Autodesk Inventor part; units mm, degrees
ref_plane "YZ Plane" through (0, 0, 0) normal (1, 0, 0) x (0, 1, 0)
ref_plane "XZ Plane" through (0, 0, 0) normal (0, 1, 0) x (-1, 0, 0)
ref_plane "XY Plane" through (0, 0, 0) normal (0, 0, 1) x (1, 0, 0)
sketch "Sketch1" plane through (0, 0, 0) normal (0, 0, 1) x (1, 0, 0)
  line L0 (27, 28) -> (27, -25)
  line L1 (27, -25) -> (-27, -25)
  line L2 (-27, -25) -> (-27, 28)
  line L3 (-30, 28) -> (-30, -28)
  line L4 (-30, -28) -> (30, -28)
  line L5 (30, -28) -> (30, 28)
  line L6 (30, 28) -> (27, 28)
  line L7 (-27, 28) -> (-30, 28)
  point P0 (0, 0)
  dimension "d4" = 56
  dimension "d5" = 53
extrude "Extrusion1" add sketch "Sketch1" along normal blind 30
sketch "Sketch2" plane through (-27, -25, 0) normal (1, 0, 0) x (0, 0, -1)
  line L0 (0, 0) -> (-30, 0)
  line L1 (0, 0) -> (0, 53)
  point P0 (0, 25)
  point P1 (-15, 45)
  dimension "d8" = 45
  dimension "d9" = 15
hole "Hole1" at (-27, 20, 15) direction (-1, 0, 0) diameter 10 end through all
sketch "Sketch3" plane through (30, -28, 0) normal (1, 0, 0) x (0, 0, -1)
  line L0 (0, 3) -> (-30, 3)
  line L1 (-30, 0) -> (-30, 56)
  point P0 (0, 28)
  point P1 (-15, 48)
  dimension "d17" = 45
  dimension "d18" = 15
hole "Hole2" at (30, 20, 15) direction (-1, 0, 0) diameter 10 end through all
sketch "Sketch4" plane through (-30, -28, 0) normal (0, -1, 0) x (1, 0, 0)
  line L0 (0, 0) -> (60, 0)
  line L1 (60, 0) -> (60, 30)
  line L2 (0, 30) -> (60, 30)
  line L3 (0, 0) -> (0, 30)
  point P0 (30, 0)
  point P1 (45, 7)
  point P2 (45, 23)
  point P3 (15, 7)
  point P4 (15, 23)
  dimension "d26" = 7
  dimension "d27" = 15
  dimension "d28" = 7
  dimension "d29" = 15
  dimension "d30" = 7
  dimension "d31" = 15
  dimension "d32" = 15
  dimension "d33" = 7
hole "Hole3" at (15, -28, 23) at (15, -28, 7) at (-15, -28, 7) at (-15, -28, 23) direction (0, 1, 0) diameter 5 end through all
fillet "Fillet1" radius 0.5 21 edges at (30, -28, 15) (30, 0, 0) (27, 1.5, 0) (0, -25, 0) (0, -28, 0) (30, 0, 30) (30, 28, 15) (0, -28, 30) (-30, -28, 15) (-27, 1.5, 0) (-27, 28, 15) (-30, 28, 15) (-30, 0, 0) (-27, 1.5, 30) (-30, 0, 30) (27, 1.5, 30) (27, 28, 15) (28.5, 28, 0) (28.5, 28, 30) (-28.5, 28, 0) (-28.5, 28, 30)
properties part number "HOLDER" material "Steel, Alloy"
The listing builds one solid part. Answer for the finished solid, in the listing's coordinates (mm). A direction names the side the tool comes from. Give positions to 0.01 mm unless a question says otherwise; leave off trailing zeros. Order: outer loops, then holes, each group sorted by start corner. A loop starts at its lowest first (then second) coordinate and runs counter-clockwise, first axis right, second up.
1) Find section B-B on y = 23. Write down the section's boundary in (x, z).
Reported:
outline: (-30, 0.5) arc R0.5 ccw to (-29.5, 0) - (-27.5, 0) arc R0.5 ccw to (-27, 0.5) - (-27, 11) - (-30, 11) - close; (-30, 19) - (-27, 19) - (-27, 29.5) arc R0.5 ccw to (-27.5, 30) - (-29.5, 30) arc R0.5 ccw to (-30, 29.5) - close; (27, 0.5) arc R0.5 ccw to (27.5, 0) - (29.5, 0) arc R0.5 ccw to (30, 0.5) - (30, 11) - (27, 11) - close; (27, 19) - (30, 19) - (30, 29.5) arc R0.5 ccw to (29.5, 30) - (27.5, 30) arc R0.5 ccw to (27, 29.5) - close
2) Given P1, Ø1.5, axis at x = -19.5, z = 15.5, coming from the +Y side, flat-ended and moving along its own axis, determine where the tip first touches the part or whether it passes through.
Reported:
P1: stops at y = -25
3) Determine the mould class of faces 3 (the face through (17.44, -26.48, 7.54)), 4 (the face through (0, -25, 15)), 5 (the face through (0, -26, 30)), 6 (the face through (0, -26, 0)) for opening direction Z: pulls with the +Z half, pulls with the -Z half, needs draft (parallel to the pull), parting line crosses it, or undercut.
Reported:
face 3: undercut
face 4: needs draft
face 5: pulls with the +Z half
face 6: pulls with the -Z half
4) Find section C-C on x = -15. Write down the section's boundary in (y, z), then the cut area to 3 significant figures.
Reported:
outline: (-28, 0.5) arc R0.5 ccw to (-27.5, 0) - (-25.5, 0) arc R0.5 ccw to (-25, 0.5) - (-25, 4.5) - (-28, 4.5) - close; (-28, 9.5) - (-25, 9.5) - (-25, 20.5) - (-28, 20.5) - close; (-28, 25.5) - (-25, 25.5) - (-25, 30) - (-27.5, 30) arc R0.5 ccw to (-28, 29.5) - close
area: 59.8 mm2
5) Consider line 1 along X through (y, z) = (-27, 23); line 2 along Z through (x, y) = (15, -25.8); line 3 along X through (y, z) = (18, 4.5). Determine where each line is inside the solid, lowest interval first.
Reported:
line 1: x = -30 to -17.5, -12.5 to 12.5, 17.5 to 30
line 2: z = 0 to 4.5, 9.5 to 20.5, 25.5 to 30
line 3: x = -30 to -27, 27 to 30
6) Find section D-D on y = -10. Write down the section's boundary in (x, z).
Reported:
outline: (-30, 0.5) arc R0.5 ccw to (-29.5, 0) - (-27.5, 0) arc R0.5 ccw to (-27, 0.5) - (-27, 29.5) arc R0.5 ccw to (-27.5, 30) - (-29.5, 30) arc R0.5 ccw to (-30, 29.5) - close; (27, 0.5) arc R0.5 ccw to (27.5, 0) - (29.5, 0) arc R0.5 ccw to (30, 0.5) - (30, 29.5) arc R0.5 ccw to (29.5, 30) - (27.5, 30) arc R0.5 ccw to (27, 29.5) - close
7) For faces 1 (the face through (27, 2, 15)), 2 (the face through (-12.78, -26.48, 5.85)), determine the directions among +Z, -Z, +X, -X, +Y, -Y from which every point of the face is accessible in a straight line to the end or side of a thin tool.
Reported:
face 1: +Z, -Z, +Y
face 2: +Y, -Y
8) Find section A-A on z = 15. Write down the section's boundary in (x, y), then the cut area to 3 significant figures.
Reported:
outline: (-30, -27.5) arc R0.5 ccw to (-29.5, -28) - (29.5, -28) arc R0.5 ccw to (30, -27.5) - (30, 15) - (27, 15) - (27, -25) - (-27, -25) - (-27, 15) - (-30, 15) - close; (-30, 25) - (-27, 25) - (-27, 27.5) arc R0.5 ccw to (-27.5, 28) - (-29.5, 28) arc R0.5 ccw to (-30, 27.5) - close; (27, 25) - (30, 25) - (30, 27.5) arc R0.5 ccw to (29.5, 28) - (27.5, 28) arc R0.5 ccw to (27, 27.5) - close
area: 438 mm2
